from build123d import *

# Parameters (mm, degrees)
F0_R     = 1.5
F1_DEPTH = 2
F2_DEPTH = 1


with BuildPart() as f1:
    # F0 (on Top) → F1 (new body)
    with BuildSketch(Plane.XY):
        with BuildLine():
            Line((12.028635, 7.386944), (-6.971365, 7.386944))
            ThreePointArc((-6.971365, 7.386944), (-9.092685, 6.508265), (-9.971365, 4.386944))
            Line((-9.971365, 4.386944), (-9.971365, -14.613056))
            ThreePointArc((-9.971365, -14.613056), (-9.092685, -16.734376), (-6.971365, -17.613056))
            Line((-6.971365, -17.613056), (12.028635, -17.613056))
            ThreePointArc((12.028635, -17.613056), (14.149955, -16.734376), (15.028635, -14.613056))
            Line((15.028635, -14.613056), (15.028635, 4.386944))
            ThreePointArc((15.028635, 4.386944), (14.149955, 6.508265), (12.028635, 7.386944))
        make_face()
        with Locations((-6.971365, 4.386944)):
            Circle(F0_R, mode=Mode.SUBTRACT)
    extrude(amount=F1_DEPTH)

    # F0 (on Top) → F2 (join)
    with BuildSketch(Plane.XY):
        with BuildLine():
            ThreePointArc((-6.971365, -17.613056), (-9.092685, -16.734376), (-9.971365, -14.613056))
            Line((-9.971365, -14.613056), (-9.971365, -22.613056))
            ThreePointArc((-9.971365, -22.613056), (-9.092685, -24.734376), (-6.971365, -25.613056))
            Line((-6.971365, -25.613056), (12.028635, -25.613056))
            ThreePointArc((12.028635, -25.613056), (14.149955, -24.734376), (15.028635, -22.613056))
            Line((15.028635, -22.613056), (15.028635, -14.613056))
            ThreePointArc((15.028635, -14.613056), (14.149955, -16.734376), (12.028635, -17.613056))
            Line((12.028635, -17.613056), (-6.971365, -17.613056))
        make_face()
    extrude(amount=F2_DEPTH)


solid = f1.part
For this review, take the finished solid that the model builds, in its own axes (mm). A direction names the side the tool comes from. Coordinates: 2 decimals unless noted, no trailing zeros. Write each loop counter-clockwise with the first axis right and the second up, starting at its lowest first coordinate (ties: lowest second). Pieces come first, ordered by that corner, then holes. Notation, with made-up numbers: (26, 26) -> (79, 26) arc R24 cw to (79, 38) -> close; hole circle Ø11 at (27.5, -21). An arc over 180 degrees is marked (long way). Write each question's results on one line, items separated by ' | '. Start each with the question number.
1) Consider section C-C (y = -17). Write out the cut boundary in (x, z).
2) Consider section D-D (x = 13). Write out the cut boundary in (y, z).
3) Consider section A-A (z = 1.5). Write out the cut boundary in (x, y), plus the area to 3 significant figures.
4) For faces 1 (the face through (2.4, -17.613, 1.5)), 2 (the face through (-9.1, 6.5, 1)), 3 (the face through (14.127, -16.758, 1.493)), 4 (the face through (-9.971, -6, 1)), 5 (the face through (-9.116, -16.711, 1.493)), list the 3-axis set-ups (+Z, -Z, +X, -X, +Y, -Y) from which the entire face can be reached by the end or side of a thin tool; tool diameter is ignored.
5) Consider section B-B (x = 4.25). Write out the cut boundary in (y, z), plus the area to 3 significant figures.
6) Insertion check: pin 1 (5.5 mm diameter, centred on x = -2, y = -22.5, fed in from +Z); pin 2 (12 mm diameter, centred on x = -2, y = -10.5, fed in from -Z); pin 3 (0.8 mm diameter, centred on x = 4.5, z = 1.5, fed in from -Y). Each pin has a flat end and moves straight along its axis. Give the tip position at first contact, or say it passes through.
7) The part is to be moulded in two halves that separate along X. For faces 6 (the face through (-8.16, 3.47, 0.99)), 7 (the face through (-9.116, -24.711, 0.493)), 8 (the face through (14.127, -24.758, 0.493)), 9 (the face through (2, -5, 2)), say which applies: +X half, -X half, draft (parallel to the pull), parting line (faces both ways), or undercut.
8) Wall thickness on L1, parallel to Y at x = -7, z = 1.15; L2, parallel to Z at x = 10, y = -22; L3, parallel to Y at x = -8.25, z = 0.5: over which ranges is each line inside the solid? List them lowest first. Write a range as [from, to].
Geometry says:
1) outline: (-9.97, 0) -> (15.03, 0) -> (15.03, 1) -> (13.85, 1) -> (13.85, 2) -> (-8.79, 2) -> (-8.79, 1) -> (-9.97, 1) -> close
2) outline: (-25.45, 0) -> (7.23, 0) -> (7.23, 2) -> (-17.45, 2) -> (-17.45, 1) -> (-25.45, 1) -> close
3) outline: (-9.97, -14.61) arc R3 ccw to (-6.97, -17.61) -> (12.03, -17.61) arc R3 ccw to (15.03, -14.61) -> (15.03, 4.39) arc R3 ccw to (12.03, 7.39) -> (-6.97, 7.39) arc R3 ccw to (-9.97, 4.39) -> close; hole circle Ø3 at (-6.97, 4.39) | area: 610 mm^2
4) face 1: +Z, +X, -X, -Y | face 2: +Z, -Z, -X, +Y | face 3: +Z, +X, -Y | face 4: +Z, -Z, -X, +Y, -Y | face 5: +Z, -X, -Y
5) outline: (-25.61, 0) -> (7.39, 0) -> (7.39, 2) -> (-17.61, 2) -> (-17.61, 1) -> (-25.61, 1) -> close | area: 58.0 mm^2
6) pin 1: z = 1 | pin 2: z = 0 | pin 3: y = -17.61
7) face 6: undercut | face 7: -X half | face 8: +X half | face 9: draft
8) L1: [-17.61, 2.89], [5.89, 7.39] | L2: [0, 1] | L3: [-25.33, 3.6], [5.17, 7.1]
